```python
from build123d import *

# Parameters (mm, degrees)
SALIENTE_EXTRUIR1_DEPTH    = 3
CROQUIS4_W                 = 3
CROQUIS4_H                 = 25
SALIENTE_EXTRUIR4_DEPTH    = 15
SALIENTE_EXTRUIR6_DEPTH    = 5
CROQUIS11_W                = 23
CROQUIS11_H                = 2
SALIENTE_EXTRUIR11_DEPTH   = 6
CROQUIS12_W                = 23
CROQUIS12_H                = 2
SALIENTE_EXTRUIR12_DEPTH   = 6
SALIENTE_EXTRUIR23_DEPTH   = 1
CROQUIS27_W                = 24
CROQUIS27_H                = 2
SALIENTE_EXTRUIR26_DEPTH   = 6
CROQUIS28_W                = 24
CROQUIS28_H                = 2
SALIENTE_EXTRUIR27_DEPTH   = 6
CROQUIS13_R                = 1.75
CORTAR_EXTRUIR1_DEPTH      = 1
CORTAR_EXTRUIR1_DEPTH_BACK = 26
REDONDEO1_R                = 3


with BuildPart() as part:
    # Croquis1 → Saliente-Extruir1 (new body)
    with BuildSketch(Plane.XY):
        with BuildLine():
            Line((79, 0), (79, 25))
            Line((79, 25), (40, 25))
            ThreePointArc((40, 25), (32, 17), (24, 25))
            Line((24, 25), (0, 25))
            Line((0, 25), (0, 0))
            Line((0, 0), (79, 0))
        make_face()
    extrude(amount=SALIENTE_EXTRUIR1_DEPTH)

    # Croquis4 → Saliente-Extruir4 (add)
    with BuildSketch(Plane(origin=(0, 0, 0), x_dir=(-1, 0, 0), z_dir=(0, 0, -1))):
        with Locations((-77.5, 12.5)):
            Rectangle(CROQUIS4_W, CROQUIS4_H)
        with Locations((-1.5, 12.5)):
            Rectangle(CROQUIS4_W, CROQUIS4_H)
    extrude(amount=SALIENTE_EXTRUIR4_DEPTH)

    # Croquis6 → Saliente-Extruir6 (add)
    with BuildSketch(Plane(origin=(0, 0, -15), x_dir=(-1, 0, 0), z_dir=(0, 0, -1))):
        with BuildLine():
            Line((-79, 25), (-79, 0))
            Line((-79, 0), (0, 0))
            Line((0, 0), (0, 25))
            Line((0, 25), (-24, 25))
            ThreePointArc((-24, 25), (-32, 17), (-40, 25))
            Line((-40, 25), (-46, 25))
            Line((-46, 25), (-46, 19))
            Line((-46, 19), (-73, 19))
            Line((-73, 19), (-73, 25))
            Line((-73, 25), (-79, 25))
        make_face()
    extrude(amount=SALIENTE_EXTRUIR6_DEPTH)

    # Croquis11 → Saliente-Extruir11 (add)
    with BuildSketch(Plane(origin=(76, 0, 0), x_dir=(0, 0, -1), z_dir=(1, 0, 0))):
        with Locations((8.5, 1)):
            Rectangle(CROQUIS11_W, CROQUIS11_H)
    extrude(amount=-SALIENTE_EXTRUIR11_DEPTH)

    # Croquis12 → Saliente-Extruir12 (add)
    with BuildSketch(Plane.ZY.offset(-3)):
        with Locations((-8.5, 1)):
            Rectangle(CROQUIS12_W, CROQUIS12_H)
    extrude(amount=-SALIENTE_EXTRUIR12_DEPTH)

    # Croquis24 → Saliente-Extruir23 (add)
    with BuildSketch(Plane(origin=(0, 0, -20), x_dir=(-1, 0, 0), z_dir=(0, 0, -1))):
        with BuildLine():
            Line((-79, 0), (-79, 25))
            Line((-79, 25), (-73, 25))
            Line((-73, 25), (-73, 19))
            Line((-73, 19), (-46, 19))
            Line((-46, 19), (-46, 25))
            Line((-46, 25), (-40, 25))
            Line((-40, 25), (-38, 25))
            ThreePointArc((-38, 25), (-32, 19), (-26, 25))
            Line((-26, 25), (0, 25))
            Line((0, 25), (0, 0))
            Line((0, 0), (-79, 0))
        make_face()
    extrude(amount=SALIENTE_EXTRUIR23_DEPTH)

    # Croquis27 → Saliente-Extruir26 (add)
    with BuildSketch(Plane(origin=(79, 0, 0), x_dir=(0, 0, -1), z_dir=(1, 0, 0))):
        with Locations((9, 24)):
            Rectangle(CROQUIS27_W, CROQUIS27_H)
    extrude(amount=SALIENTE_EXTRUIR26_DEPTH)

    # Croquis28 → Saliente-Extruir27 (add)
    with BuildSketch(Plane.ZY):
        with Locations((-9, 24)):
            Rectangle(CROQUIS28_W, CROQUIS28_H)
    extrude(amount=SALIENTE_EXTRUIR27_DEPTH)

    # Croquis13 → Cortar-Extruir1 (cut, two sides)
    with BuildSketch(Plane(origin=(0, 25, 0), x_dir=(1, 0, 0), z_dir=(0, 1, 0))) as cortar_extruir1_sk:
        with Locations((82, 15)):
            Circle(CROQUIS13_R)
        with Locations((82, 3)):
            Circle(CROQUIS13_R)
        with Locations((73, 11)):
            Circle(CROQUIS13_R)
        with Locations((73, 4)):
            Circle(CROQUIS13_R)
        with Locations((6, 4)):
            Circle(CROQUIS13_R)
        with Locations((6, 11)):
            Circle(CROQUIS13_R)
        with Locations((-3, 3)):
            Circle(CROQUIS13_R)
        with Locations((-3, 15)):
            Circle(CROQUIS13_R)
    extrude(amount=CORTAR_EXTRUIR1_DEPTH, mode=Mode.SUBTRACT)
    extrude(cortar_extruir1_sk.sketch, amount=-CORTAR_EXTRUIR1_DEPTH_BACK, mode=Mode.SUBTRACT)

    # Redondeo1
    redondeo1_edges = [part.edges().sort_by_distance(p)[0] for p in [
        (46, 19, -18),
        (73, 19, -18),
    ]]
    fillet(redondeo1_edges, radius=REDONDEO1_R)


solid = part.part
```
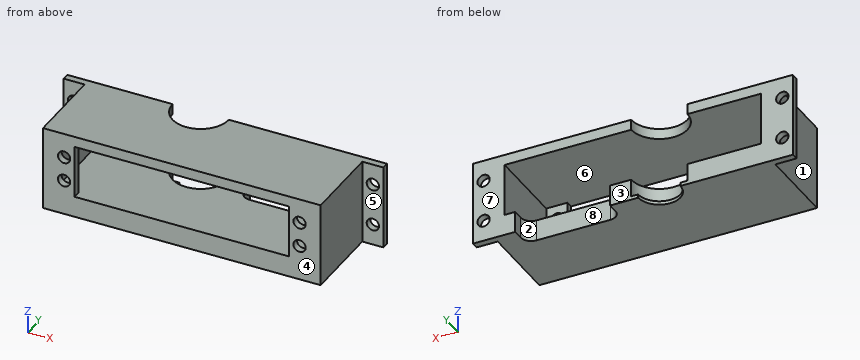
Design review of the part built by this model. Coordinates are the model's own, in mm. Face numbers are marked on the shaded views. A direction names the side the tool comes from. Coordinates: 2 decimals unless noted, no trailing zeros. Write each loop counter-clockwise with the first axis right and the second up, starting at its lowest first coordinate (ties: lowest second). Pieces come first, ordered by that corner, then holes.
1) To check wall thickness, follow L1, parallel to Z at x = 73, y = 1.15; L2, parallel to X at y = 0.5, z = -4; L3, parallel to X at y = 23.5, z = -3. State the ranges of each line that lie inside material, in increasing order.
2) Add section B-B (x = 6). Write out the cut boundary in (y, z).
3) Insertion check: pin 1 (3 mm diameter, centred on x = 7, z = -10.5, fed in from +Y); pin 2 (4 mm diameter, centred on y = 18, z = -13, fed in from -X); pin 3 (0.6 mm diameter, centred on y = 1, z = -7, fed in from +X). Each pin has a flat end and moves straight along its axis. Give the tip position at first contact, or say it passes through.
4) Add section A-A (x = 53.5). Write out the cut boundary in (y, z).
5) Machinability: for the marked faces 4, 5, 6, 7 and 8, which of the approach directions +Z, -Z, +X, -X, +Y, -Y give a long, thin tool a straight path to every point of the face, cutting with its end or side? Answer none if there is none.
6) Mouldability with a two-part tool opening along X and no side actions: class the marked faces 1, 2 and 3 as +X half, -X half, draft (parallel to the pull), parting line (faces both ways), or undercut.
7) Add section C-C (y = 4). Write out the cut boundary in (x, z).
8) Add section D-D (x = 18). Write out the cut boundary in (y, z).
Check result:
1. L1: z = -21 to -12.75, -9.25 to -5.75, -2.25 to 3
1. L2: x = 0 to 4.25, 7.75 to 9, 70 to 71.25, 74.75 to 79
1. L3: x = -6 to -4.75, -1.25 to 3, 76 to 80.25, 83.75 to 85
2. outline: (0, -21) - (25, -21) - (25, -15) - (2, -15) - (2, -12.75) - (0, -12.75) - close; (0, -9.25) - (2, -9.25) - (2, -5.75) - (0, -5.75) - close; (0, -2.25) - (2, -2.25) - (2, 0) - (25, 0) - (25, 3) - (0, 3) - close
3. pin 1: stops at y = 2
3. pin 2: stops at x = 0
3. pin 3: stops at x = 79
4. outline: (0, -21) - (19, -21) - (19, -15) - (0, -15) - close; (0, 0) - (25, 0) - (25, 3) - (0, 3) - close
5. face 4: +Z, -Z, +X, -X, -Y
5. face 5: +Z, -Z, +X, -Y
5. face 6: +Y
5. face 7: +Z, -Z, +X, -X, +Y
5. face 8: -Z, +Y
6. face 1: -X half
6. face 2: undercut
6. face 3: draft
7. outline: (0, -21) - (79, -21) - (79, 3) - (0, 3) - close; hole (3, -15) - (76, -15) - (76, 0) - (3, 0) - close
8. outline: (0, -21) - (25, -21) - (25, -15) - (0, -15) - close; (0, 0) - (25, 0) - (25, 3) - (0, 3) - close
